```python
from build123d import *

# Parameters (mm, degrees)
SKETCH1_W           = 3.937
SKETCH1_H           = 2.54
BOSS_EXTRUDE1_DEPTH = 15.875


with BuildPart() as part:
    # Sketch1 → Boss-Extrude1 (new body)
    with BuildSketch(Plane(origin=(0, 0, 0), x_dir=(1, 0, 0), z_dir=(0, 1, 0))):
        Polygon((4.0005, 2.54), (-4.0005, 2.54), (-4.0005, 0), (-4.0005, -9.525), (-1.4605, -9.525), (-1.4605, 0), (1.4605, 0), (1.4605, -9.525), (4.0005, -9.525), (4.0005, 0), align=None)
        with Locations((-5.969, 1.27)):
            Rectangle(SKETCH1_W, SKETCH1_H)
        with Locations((5.969, 1.27)):
            Rectangle(SKETCH1_W, SKETCH1_H)
    extrude(amount=BOSS_EXTRUDE1_DEPTH)


solid = part.part
```
Geometry: final body of the model. Coordinates: model frame, mm. A direction names the side the tool comes from. Round coordinates to 2 decimals unless told otherwise and drop trailing zeros. Write each loop counter-clockwise with the first axis right and the second up, starting at its lowest first coordinate (ties: lowest second). Pieces come first, ordered by that corner, then holes. Notation, with made-up numbers: (-19, 29.5) -> (16, 29.5) arc R31 ccw to (16, 53.5) -> close; hole circle Ø5 at (-38, 48). An arc over 180 degrees is marked (long way). Use CSV: the item, a comma, the result in double quotes. Start each with the question number.
Q1. Line query: L1, parallel to X at y = 11.5, z = 6.5; L2, parallel to Z at x = -1.25, y = 10. Output: solid intervals per line, ascending.
Q2. First-contact query: pin 1 Ø3 at (y, z) = (4, 4) entering from -X; pin 2 Ø5 at (x, y) = (5.5, 9) entering from +Z (3 decimals); pin 3 Ø1.2 at (x, y) = (-5.5, 6) entering from +Z; pin 4 Ø3 at (y, z) = (13, 2.5) entering from +X. Flat tips, straight axial feed; report the tip coordinate or a pass-through.
Q3. Reachability of faces 4 (the face through (1.46, 8, 5)), 5 (the face through (-6, 8, 0)), 6 (the face through (-7.938, 8, -1)), 7 (the face through (4, 8, 5)) from +Z, -Z, +X, -X, +Y, -Y: full face, straight path, thin tool, end or side. Return the list, or none.
Q4. Section B-B (y = 3). Return loops of the section in (x, z) (1 decimal).
Q5. Section A-A (z = 2.5). Return loops of the section in (x, y) (1 decimal), plus the area to 3 significant figures.
Q6. Pull-direction query (X, two-part tool) for faces 1 (the face through (7.938, 8, -1)), 2 (the face through (-1.46, 8, 5)), 3 (the face through (3, 8, 9.525)); classes: pulls with the +X half, pulls with the -X half, needs draft (parallel to the pull), parting line crosses it, or undercut.
Q7. Section C-C (x = 5.75). Return loops of the section in (y, z) (3 decimals), plus the area to 3 significant figures.
Result sheet:
1,L1,"-4 to -1.46, 1.46 to 4"
1,L2,"-2.54 to 0"
2,pin 1,"x = -4"
2,pin 2,"z = 9.525"
2,pin 3,"z = 0"
2,pin 4,"x = 4"
3,face 4,"+Z, +Y, -Y"
3,face 5,"+Z, -X, +Y, -Y"
3,face 6,"+Z, -Z, -X, +Y, -Y"
3,face 7,"+Z, +X, +Y, -Y"
4,outline,"(-7.9, -2.5) -> (7.9, -2.5) -> (7.9, 0) -> (4, 0) -> (4, 9.5) -> (1.5, 9.5) -> (1.5, 0) -> (-1.5, 0) -> (-1.5, 9.5) -> (-4, 9.5) -> (-4, 0) -> (-7.9, 0) -> close"
5,outline,"(-4, 0) -> (-1.5, 0) -> (-1.5, 15.9) -> (-4, 15.9) -> close; (1.5, 0) -> (4, 0) -> (4, 15.9) -> (1.5, 15.9) -> close"
5,area,"80.6 mm²"
6,face 1,"pulls with the +X half"
6,face 2,"undercut"
6,face 3,"needs draft"
7,outline,"(0, -2.54) -> (15.875, -2.54) -> (15.875, 0) -> (0, 0) -> close"
7,area,"40.3 mm²"
